from build123d import *

# Parameters (mm, degrees)
SKETCH2_W                = 66
SKETCH2_H                = 30
BOSS_EXTRUDE1_DEPTH      = 58
SKETCH3_R                = 9
SKETCH3_R_2              = 7.5
BOSS_EXTRUDE2_DEPTH      = 2
SKETCH4_R                = 2.5
BOSS_EXTRUDE3_DEPTH      = 10
BOSS_EXTRUDE4_DEPTH      = 1
BOSS_EXTRUDE4_DEPTH_BACK = 5
SKETCH5_R                = 27.5
SKETCH6_W                = 6
SKETCH6_H                = 20
BOSS_EXTRUDE5_DEPTH      = 3
SKETCH7_R                = 1
BOSS_EXTRUDE6_DEPTH      = 3


with BuildPart() as part:
    # Sketch2 → Boss-Extrude1 (new body)
    with BuildSketch(Plane(origin=(0, 0, 0), x_dir=(1, 0, 0), z_dir=(0, 1, 0))):
        with Locations((-46.568123526, -34.860945828)):
            Rectangle(SKETCH2_W, SKETCH2_H)
    extrude(amount=BOSS_EXTRUDE1_DEPTH)

    # Sketch3 → Boss-Extrude2 (add)
    with BuildSketch(Plane(origin=(0, 58, 0), x_dir=(1, 0, 0), z_dir=(0, 1, 0))):
        with Locations(Location((-63.068123526, -34.860945828, 0), (0, 0, 270))):
            Circle(SKETCH3_R)
        with Locations(Location((-63.068123526, -34.860945828, 0), (0, 0, 270))):
            Circle(SKETCH3_R_2, mode=Mode.SUBTRACT)
    extrude(amount=BOSS_EXTRUDE2_DEPTH)

    # Sketch4 → Boss-Extrude3 (add)
    with BuildSketch(Plane(origin=(0, 58, 0), x_dir=(1, 0, 0), z_dir=(0, 1, 0))):
        with Locations(Location((-63.068123526, -34.860945828, 0), (0, 0, 270))):
            Circle(SKETCH4_R)
    extrude(amount=BOSS_EXTRUDE3_DEPTH)

    # Sketch5 → Boss-Extrude4 (add, two sides: drawn at the far end of the back side and taken through both)
    with BuildSketch(Plane(origin=(0, 68, 0), x_dir=(1, 0, 0), z_dir=(0, 1, 0)).offset(-BOSS_EXTRUDE4_DEPTH_BACK)):
        with Locations(Location((-63.068123526, -34.860945828, 0), (0, 0, 270))):
            Circle(SKETCH5_R)
    extrude(amount=BOSS_EXTRUDE4_DEPTH + BOSS_EXTRUDE4_DEPTH_BACK)

    # Sketch6 → Boss-Extrude5 (add)
    with BuildSketch(Plane.XZ):
        with Locations((-66.568123526, 34.860945828)):
            Rectangle(SKETCH6_W, SKETCH6_H)
    extrude(amount=BOSS_EXTRUDE5_DEPTH)

    # Sketch7 → Boss-Extrude6 (add)
    with BuildSketch(Plane.XZ.offset(3)):
        with Locations(Location((-66.568123526, 29.860945828, 0), (0, 0, 90))):
            Circle(SKETCH7_R)
        with Locations(Location((-66.568123526, 39.860945828, 0), (0, 0, 90))):
            Circle(SKETCH7_R)
    extrude(amount=BOSS_EXTRUDE6_DEPTH)


solid = part.part
Input: part model. Units: mm. Frame: model coordinates. A direction names the side the tool comes from. Coordinates: 2 decimals unless noted, no trailing zeros. Write each loop counter-clockwise with the first axis right and the second up, starting at its lowest first coordinate (ties: lowest second). Pieces come first, ordered by that corner, then holes. Notation, with made-up numbers: M -33,58.5 L 21,58.5 A30 cw 21,84.5 Z; hole C -10.75,77.5 d1. An arc over 180 degrees is marked long. Answer as a JSON object with one key per item and string values. Group by question number.
(1) Ray query, line 1 along Y through (x, z) = (-72, 31); line 2 along Z through (x, y) = (-41.5, 1); line 3 along Y through (x, z) = (-33.5, 36). Return the intervals inside material, ascending. Write a range as [from, to].
(2) Section A-A on z = 21. Output: boundary loops of the cut face in (x, y).
(3) Section C-C on y = 11.5. Output: boundary loops of the cut face in (x, z), plus the area to 3 significant figures.
(4) Contact query for flat-ended pins moving along their axis: P1, Ø2.5, axis at y = -1.5, z = 33.5, coming from the +X side; P2, Ø0.9, axis at x = -66.5, y = -1, coming from the -Z side; P3, Ø9, axis at x = -43.5, z = 37, coming from the -Y side. Output: stop coordinate, or through.
(5) Section D-D on x = -28. Output: boundary loops of the cut face in (y, z).
(6) Set-up query: faces 5 (the face through (-39.88, 65.958, 49.645)), 6 (the face through (-71.053, 58.986, 39.014)), 7 (the face through (-47, 29, 49.861)), 8 (the face through (-67, -1, 24.861)). Return all of +Z, -Z, +X, -X, +Y, -Y with unobstructed straight access to the full face (end or side cutting, diameter ignored); none if empty.
(7) Mould query, pull axis Z, two halves, no side actions, for faces 1 (the face through (-67, -1, 44.861)), 2 (the face through (-64.59, 60.46, 32.88)), 3 (the face through (-66.61, -4.48, 28.86)), 4 (the face through (-56, 60, 31)). Classes: pulls with the +Z half, pulls with the -Z half, needs draft (parallel to the pull), parting line crosses it, or undercut.
(8) Section B-B on z = 33.5. Output: boundary loops of the cut face in (x, y), plus the area to 3 significant figures.
Result set:
{
 "1": {"line 1": "y = [0, 58], [63, 69]", "line 2": "z = [19.86, 49.86]", "line 3": "y = [0, 58]"},
 "2": {"outline": "M -86.82,63 L -39.32,63 L -39.32,69 L -86.82,69 Z; M -79.57,0 L -13.57,0 L -13.57,58 L -79.57,58 Z"},
 "3": {"outline": "M -79.57,19.86 L -13.57,19.86 L -13.57,49.86 L -79.57,49.86 Z", "area": "1,980 mm2"},
 "4": {"P1": "stops at x = -63.57", "P2": "stops at z = 24.86", "P3": "stops at y = 0"},
 "5": {"outline": "M 0,19.86 L 58,19.86 L 58,49.86 L 0,49.86 Z"},
 "6": {"face 5": "+Y", "face 6": "none", "face 7": "+Z, +X, -X, -Y", "face 8": "-Z, +X, -X, -Y"},
 "7": {"face 1": "pulls with the +Z half", "face 2": "undercut", "face 3": "undercut", "face 4": "needs draft"},
 "8": {"outline": "M -90.53,63 L -65.17,63 L -65.17,58 L -70.44,58 L -70.44,60 L -71.96,60 L -71.96,58 L -79.57,58 L -79.57,0 L -69.57,0 L -69.57,-3 L -63.57,-3 L -63.57,0 L -13.57,0 L -13.57,58 L -54.17,58 L -54.17,60 L -55.69,60 L -55.69,58 L -60.97,58 L -60.97,63 L -35.6,63 L -35.6,69 L -90.53,69 Z", "area": "4,200 mm2"}
}
